Part model, mm, in its own coordinate system. Face numbers are marked on the shaded views. A direction names the side the tool comes from. Round coordinates to 2 decimals unless told otherwise and drop trailing zeros. Order: outer loops, then holes, each group sorted by start corner. A loop starts at its lowest first (then second) coordinate and runs counter-clockwise, first axis right, second up. Notation, with made-up numbers: (24, 39.25) -> (38, 39.25) arc R25 cw to (38, 70.25) -> close; hole circle Ø11 at (82, 52.25). An arc over 180 degrees is marked (long way). Use CSV: the item, a comma, the result in double quotes.
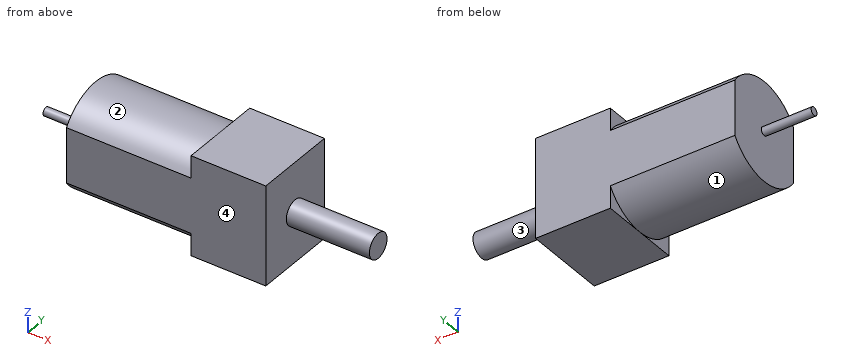
```python
from build123d import *

# Parameters (mm, degrees)
SKETCH2_W           = 12
SKETCH2_H           = 10
BOSS_EXTRUDE1_DEPTH = 24
SKETCH3_R           = 1.5
BOSS_EXTRUDE2_DEPTH = 10
SKETCH4_OUTSIDE_W   = 21.484
SKETCH4_OUTSIDE_H   = 19.484
SKETCH4_OUTSIDE_R   = 6
CUT_EXTRUDE1_DEPTH  = 15
SKETCH5_R           = 0.5
BOSS_EXTRUDE3_DEPTH = 6


with BuildPart() as part:
    # Sketch2 → Boss-Extrude1 (new body)
    with BuildSketch(Plane(origin=(0, 0, 0), x_dir=(0, 0, -1), z_dir=(1, 0, 0))):
        with Locations((6, 5)):
            Rectangle(SKETCH2_W, SKETCH2_H)
    extrude(amount=BOSS_EXTRUDE1_DEPTH)

    # Sketch3 → Boss-Extrude2 (add)
    with BuildSketch(Plane(origin=(24, 0, 0), x_dir=(0, 0, -1), z_dir=(1, 0, 0))):
        with Locations(Location((6, 5, 0), (0, 0, 180))):
            Circle(SKETCH3_R)
    extrude(amount=BOSS_EXTRUDE2_DEPTH)

    # Sketch4 outside → Cut-Extrude1 (cut)
    with BuildSketch(Plane.ZY):
        with Locations((-6, 5)):
            Rectangle(SKETCH4_OUTSIDE_W, SKETCH4_OUTSIDE_H)
        with Locations((-6, 5)):
            Circle(SKETCH4_OUTSIDE_R, mode=Mode.SUBTRACT)
    extrude(amount=-CUT_EXTRUDE1_DEPTH, mode=Mode.SUBTRACT)

    # Sketch5 → Boss-Extrude3 (add)
    with BuildSketch(Plane.ZY):
        with Locations((-6, 5)):
            Circle(SKETCH5_R)
    extrude(amount=BOSS_EXTRUDE3_DEPTH)


solid = part.part
```
(1) Cut at C-C, the plane x = 9.5. Give the cut face in (y, z).
Reply:
outline,"(0, -9.32) arc R6 ccw to (10, -9.32) -> (10, -2.68) arc R6 ccw to (0, -2.68) -> close"
(2) Drop flat-ended pins along their axis: P1, Ø1.3, axis at y = 3, z = -10, coming from the -X side; P2, Ø4, axis at x = 7, y = 8, coming from the +Z side. Give the stop position or say it passes through.
Reply:
P1,"x = 0"
P2,"z = -0.08"
(3) Cut at D-D, the plane x = 28. Give the cut face in (y, z), then the cut area to 3 significant figures.
Reply:
outline,"circle Ø3 at (5, -6)"
area,"7.07 mm2"
(4) Cut at A-A, the plane z = -6. Give the cut face in (x, y).
Reply:
outline,"(-6, 4.5) -> (0, 4.5) -> (0, 0) -> (24, 0) -> (24, 3.5) -> (34, 3.5) -> (34, 6.5) -> (24, 6.5) -> (24, 10) -> (0, 10) -> (0, 5.5) -> (-6, 5.5) -> close"
(5) Probe probe 1 along X at (y, z) = (8.5, -6); probe 2 along Z at (x, y) = (10.5, 6); probe 3 along Z at (x, y) = (5.5, 7.75). List the from-to ranges inside material, lowest first. Write a range as [from, to].
Reply:
probe 1,"[0, 24]"
probe 2,"[-11.92, -0.08]"
probe 3,"[-11.33, -0.67]"
(6) Which spindle directions (+Z, -Z, +X, -X, +Y, -Y) get a long thin tool onto all of the face, cutting with end or side? Do the marked faces 1, 2, 3 and 4. Say none if no direction does.
Reply:
face 1,"-Z, -X"
face 2,"+Z, -X"
face 3,"+X"
face 4,"+Z, -Z, +X, -X, -Y"
(7) Cut at B-B, the plane y = 6. Give the cut face in (x, z), then the cut area to 3 significant figures.
Reply:
outline,"(0, -11.92) -> (15, -11.92) -> (15, -12) -> (24, -12) -> (24, -7.12) -> (34, -7.12) -> (34, -4.88) -> (24, -4.88) -> (24, 0) -> (15, 0) -> (15, -0.08) -> (0, -0.08) -> close"
area,"308 mm2"
